Autodesk Inventor part; units mm, degrees
ref_plane "YZ Plane" through (0, 0, 0) normal (1, 0, 0) x (0, 1, 0)
ref_plane "XZ Plane" through (0, 0, 0) normal (0, 1, 0) x (-1, 0, 0)
ref_plane "XY Plane" through (0, 0, 0) normal (0, 0, 1) x (1, 0, 0)
sketch "Esboço1" plane through (0, 0, 0) normal (0, 0, 1) x (1, 0, 0)
  line L0 (0, 0) -> (9, 0)
  line L1 (9, 0) -> (9, 3.5)
  line L2 (9, 3.5) -> (0, 3.5)
  line L3 (0, 3.5) -> (0, 0)
  line L4 (9, 3.5) -> (9.6171, 0)
  line L5 (9.6171, 0) -> (9, 0)
  line L6 (9.6171, 0) -> (187.8673, 31.4303)
  line L7 (9, 3.5) -> (187.2502, 34.9303)
  line L8 (187.8673, 31.4303) -> (187.2502, 34.9303)
  point P0 (0, 1.75)
  point P1 (4.5, 0)
  dimension "d0" = 3.5
  dimension "d1" = 10
  dimension "d2" = 181
  dimension "d17" = 9
extrude "Extrusão1" add sketch "Esboço1" along normal mid plane 7
sketch "Esboço4" plane through (0, 0, 0) normal (0, 0, 1) x (1, 0, 0)
  line L0 (187.2502, 34.9303) -> (9, 3.5)
  line L1 (9, 3.5) -> (0, 3.5)
  line L2 (187.7711, 31.9759) -> (9.2625, 0.5)
  line L3 (9.2625, 0.5) -> (0, 0.5)
  line L4 (187.7711, 31.9759) -> (187.2502, 34.9303)
  line L5 (0, 0.5) -> (0, 3.5)
  point P0 (0, 0)
  dimension "d13" = 3
extrude "Extrusão4" cut sketch "Esboço4" along normal mid plane 6
fillet "Arredondamento1" radius 3 4 edges at (98.5168, 16.2379, 3) (4.6312, 0.5, 3) (4.6312, 0.5, -3) (98.5168, 16.2379, -3)
properties part number "Inverter sentido bolinha"
Source: CAD feature listing. Evaluate the final solid. Frame: model axes, mm. A direction names the side the tool comes from. Coordinates: 2 decimals unless noted, no trailing zeros. Loops run counter-clockwise (first coordinate to the right, second up) from the corner with the lowest first, then second, coordinate; pieces in that order, holes last. Notation, with made-up numbers: M 24.5,83 L 83.5,83 A14 cw 83.5,91 Z; hole C 65.25,81.25 d2. An arc over 180 degrees is marked long. Use a Markdown table: item, result. Add a question column.
Q1. Material intervals for L1, parallel to Z at x = 105, y = 19; L2, parallel to Z at x = 9, y = 2.5; L3, parallel to Y at x = 176.5, z = 2.5, sorted ascending.
Q2. Access query for faces 4 (the flat face through (96.9, 19, -3.3)), 5 (the cylindrical face through (4.57, 1.4, -2.14)). Directions: +Z, -Z, +X, -X, +Y, -Y. A direction counts if a zero-diameter tool reaches every point of the face in a straight line with its end or side. Return the directions, or none.
Q3. Draft query along Z for faces 1 (the flat face through (93, 16, 3.5)), 2 (the cylindrical face through (97.111, 16.906, -2.145)), 3 (the flat face through (0, 0.2, 0)). Return one class per face: pulls with the +Z half, pulls with the -Z half, needs draft (parallel to the pull), parting line crosses it, or undercut.
Q4. Section query A-A, the plane z = 1.5. Return loops of the section in (x, y).
Q5. First-contact query: pin 1 (15.5 mm diameter, centred on x = 95.5, y = 12.5, fed in from -Z); pin 2 (3 mm diameter, centred on x = 152, z = -2.5, fed in from +Y). Flat tips, straight axial feed; report the tip coordinate or a pass-through.
Result:
| question | item | result |
|---|---|---|
| 1 | L1 | z = -3.5 to -2.65, 2.65 to 3.5 |
| 1 | L2 | z = -3.5 to -2.83, 2.83 to 3.5 |
| 1 | L3 | y = 29.43 to 31.35 |
| 2 | face 4 | +Z, -Z, -X, +Y |
| 2 | face 5 | -X, +Y |
| 3 | face 1 | pulls with the +Z half |
| 3 | face 2 | undercut |
| 3 | face 3 | needs draft |
| 4 | outline | M 0,0 L 9.62,0 L 187.87,31.43 L 187.7,32.37 L 9.23,0.9 L 0,0.9 Z |
| 5 | pin 1 | stops at z = -3.5 |
| 5 | pin 2 | stops at y = 28.96 |
